The listing builds one solid part. Answer for the finished solid, in the listing's coordinates (mm). A direction names the side the tool comes from. Round coordinates to 2 decimals unless told otherwise and drop trailing zeros. Loops run counter-clockwise (first coordinate to the right, second up) from the corner with the lowest first, then second, coordinate; pieces in that order, holes last. Notation, with made-up numbers: M -19,24.25 L 24,24.25 A7 ccw 24,35.25 Z; hole C -12.75,-37.5 d9. An arc over 180 degrees is marked long. Answer as a JSON object with one key per item and string values.
Autodesk Inventor part; units mm, degrees
ref_plane "YZ Plane" through (0, 0, 0) normal (1, 0, 0) x (0, 1, 0)
ref_plane "XZ Plane" through (0, 0, 0) normal (0, 1, 0) x (-1, 0, 0)
ref_plane "XY Plane" through (0, 0, 0) normal (0, 0, 1) x (1, 0, 0)
sketch "Sketch1" plane through (0, 0, 0) normal (0, 1, 0) x (-1, 0, 0)
  line L0 (0, 0) -> (-25.4, 0)
  line L1 (-25.4, 0) -> (-25.4, -25.4)
  line L2 (-25.4, -25.4) -> (0, -25.4)
  line L3 (0, -25.4) -> (0, 0)
  line L4 (-1.5875, -23.8125) -> (-23.8125, -23.8125)
  line L5 (-23.8125, -23.8125) -> (-23.8125, -1.5875)
  line L6 (-23.8125, -1.5875) -> (-1.5875, -1.5875)
  line L7 (-1.5875, -1.5875) -> (-1.5875, -23.8125)
  dimension "d0" = 25.4
  dimension "d1" = 25.4
  dimension "d2" = 1.5875
extrude "Extrusion1" add sketch "Sketch1" along normal blind 342.9
sketch "Sketch2" plane through (0, 0, 0) normal (0, 0, 1) x (1, 0, 0)
  line L0 (0, 342.9) -> (25.4, 342.9)
  line L1 (0, 0) -> (0, 342.9)
  point P0 (12.7, 298.45)
  dimension "d5" = 44.45
  dimension "d6" = 12.7
hole "Hole1" at (12.7, 298.45, 0) direction (0, 0, -1) diameter 6.35 end through all
sketch "Sketch3" plane through (0, 0, 0) normal (0, 0, 1) x (1, 0, 0)
  line L0 (0, 342.9) -> (25.4, 342.9)
  line L1 (0, 0) -> (0, 342.9)
  point P0 (12.7, 254)
  dimension "d14" = 88.9
  dimension "d15" = 12.7
hole "Hole2" at (12.7, 254, 0) direction (0, 0, -1) diameter 6.35 end through all
properties part number "gripper main arm"
Item 1: Which of the six approach directions +Z, -Z, +X, -X, +Y, -Y give full straight-line access (tool end or side, diameter ignored) to faces 1 (the face through (24, 0, -13)), 2 (the face through (1.588, 169, -13))?
Values follow:
{"face 1": "+Z, -Z, +X, -X, -Y", "face 2": "+Y, -Y"}
Item 2: Determine the mould class of faces 3 (the face through (0, 169, -13)), 4 (the face through (13, 169, -25.4)), 5 (the face through (13, 169, -23.812)) for opening direction Z: released by +Z, released by -Z, zero draft, split by the parting line, or undercut.
Values follow:
{"face 3": "zero draft", "face 4": "released by -Z", "face 5": "undercut"}
Item 3: The part is cut by section B-B (z = -18.75). Give the vertices of the cut face in (x, y).
Values follow:
{"outline": "M 0,0 L 1.59,0 L 1.59,342.9 L 0,342.9 Z; M 23.81,0 L 25.4,0 L 25.4,342.9 L 23.81,342.9 Z"}
Item 4: The part is cut by section D-D (y = 69). Give the vertices of the cut face in (x, z).
Values follow:
{"outline": "M 0,-25.4 L 25.4,-25.4 L 25.4,0 L 0,0 Z; hole M 1.59,-23.81 L 23.81,-23.81 L 23.81,-1.59 L 1.59,-1.59 Z"}
Item 5: The part is cut by section C-C (y = 298.45). Give the vertices of the cut face in (x, z) (1 decimal), then the cut area to 3 significant figures.
Values follow:
{"outline": "M 0,-25.4 L 9.5,-25.4 L 9.5,-23.8 L 1.6,-23.8 L 1.6,-1.6 L 9.5,-1.6 L 9.5,0 L 0,0 Z; M 15.9,-25.4 L 25.4,-25.4 L 25.4,0 L 15.9,0 L 15.9,-1.6 L 23.8,-1.6 L 23.8,-23.8 L 15.9,-23.8 Z", "area": "131 mm^2"}
Item 6: Straight lines are drawn through the part: line 1 (Y direction, x = 12.7, z = -24.4) (3 decimals); line 2 (Z direction, x = 3.5, y = 259.5); line 3 (X direction, y = 45, z = -23.75). For each, find the intervals that lie inside material, in ascending order.
Values follow:
{"line 1": "0 to 250.825, 257.175 to 295.275, 301.625 to 342.9", "line 2": "-25.4 to -23.81, -1.59 to 0", "line 3": "0 to 1.59, 23.81 to 25.4"}
Item 7: The part is cut by section A-A (x = 19.5). Give the vertices of the cut face in (y, z).
Values follow:
{"outline": "M 0,-25.4 L 342.9,-25.4 L 342.9,-23.81 L 0,-23.81 Z; M 0,-1.59 L 342.9,-1.59 L 342.9,0 L 0,0 Z"}
